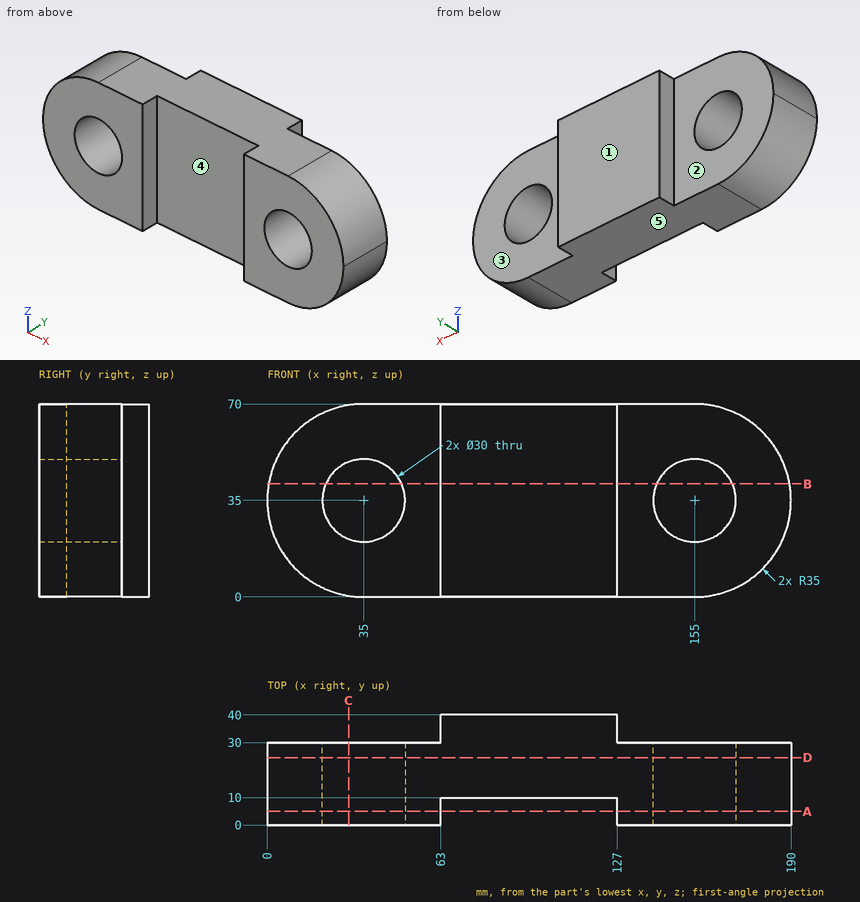
Could you check a few things on this drawing? It's one solid part, dimensions in mm from its lowest x, y, z. A direction names the side the tool comes from. Give positions to 0.01 mm unless a question says otherwise; leave off trailing zeros. Write each loop counter-clockwise with the first axis right and the second up, starting at its lowest first coordinate (ties: lowest second). Pieces come first, ordered by that corner, then holes. Notation, with made-up numbers: (-14, -28.75) -> (16, -28.75) arc R17 cw to (16, -13.75) -> close; hole circle Ø5 at (40, -10.75). An arc over 180 degrees is marked (long way). Answer as a JSON object with one key per item and string values.
Q1. Please list where these lines run through material, in increasing order: L1, parallel to Z at x = 155, y = 6; L2, parallel to Y at x = 177.5, z = 29.5; L3, parallel to X at y = 23, z = 25.
Taken from the geometry:
{"L1": "z = 0 to 20, 50 to 70", "L2": "y = 0 to 30", "L3": "x = 1.46 to 23.82, 46.18 to 143.82, 166.18 to 188.54"}
Q2. Suppose I cut it at B-B on z = 41. Write out the boundary of the cut face in (x, y).
Taken from the geometry:
{"outline": "(0.52, 0) -> (21.25, 0) -> (21.25, 30) -> (0.52, 30) -> close; (48.75, 0) -> (63, 0) -> (63, 10) -> (127, 10) -> (127, 0) -> (141.25, 0) -> (141.25, 30) -> (127, 30) -> (127, 40) -> (63, 40) -> (63, 30) -> (48.75, 30) -> close; (168.75, 0) -> (189.48, 0) -> (189.48, 30) -> (168.75, 30) -> close"}
Q3. Suppose I cut it at A-A on y = 5. Write out the boundary of the cut face in (x, z).
Taken from the geometry:
{"outline": "(35, 0) -> (63, 0) -> (63, 70) -> (35, 70) arc R35 ccw to start; (127, 0) -> (155, 0) arc R35 ccw to (155, 70) -> (127, 70) -> close; hole circle Ø30 at (35, 35); hole circle Ø30 at (155, 35)"}
Q4. Suppose I cut it at D-D on y = 24.5. Write out the boundary of the cut face in (x, z), then the cut area to 3 significant figures.
Taken from the geometry:
{"outline": "(35, 0) -> (155, 0) arc R35 ccw to (155, 70) -> (35, 70) arc R35 ccw to start; hole circle Ø30 at (35, 35); hole circle Ø30 at (155, 35)", "area": "10,800 mm²"}
Q5. Which directions (+Z, -Z, +X, -X, +Y, -Y) give clear straight access to the entire face, cutting with the end or side of a thin tool? Please do the marked faces 1, 2 and 3.
Taken from the geometry:
{"face 1": "+Z, -Z, +X, -X, +Y", "face 2": "+Z, -Z, -X, +Y", "face 3": "+Z, -Z, +X, +Y"}
Q6. Suppose I cut it at C-C on x = 29.5. Write out the boundary of the cut face in (y, z), then the cut area to 3 significant figures.
Taken from the geometry:
{"outline": "(0, 0.43) -> (30, 0.43) -> (30, 21.04) -> (0, 21.04) -> close; (0, 48.96) -> (30, 48.96) -> (30, 69.57) -> (0, 69.57) -> close", "area": "1,240 mm²"}
Q7. Will these pins go through, and if not, where does the flat tip stop? pin 1 Ø3 at (y, z) = (11, 16.5) entering from -X; pin 2 Ø11 at (y, z) = (6.5, 47.5) entering from -X; pin 3 Ø8 at (y, z) = (4, 25.5) entering from +X.
Taken from the geometry:
{"pin 1": "stops at x = 4.41", "pin 2": "stops at x = 0.71", "pin 3": "stops at x = 189.57"}
Q8. We'd pull the mould along X, two halves only. Please class the marked faces 4 and 5: released by +X, released by -X, zero draft, split by the parting line, or undercut.
Taken from the geometry:
{"face 4": "undercut", "face 5": "zero draft"}
